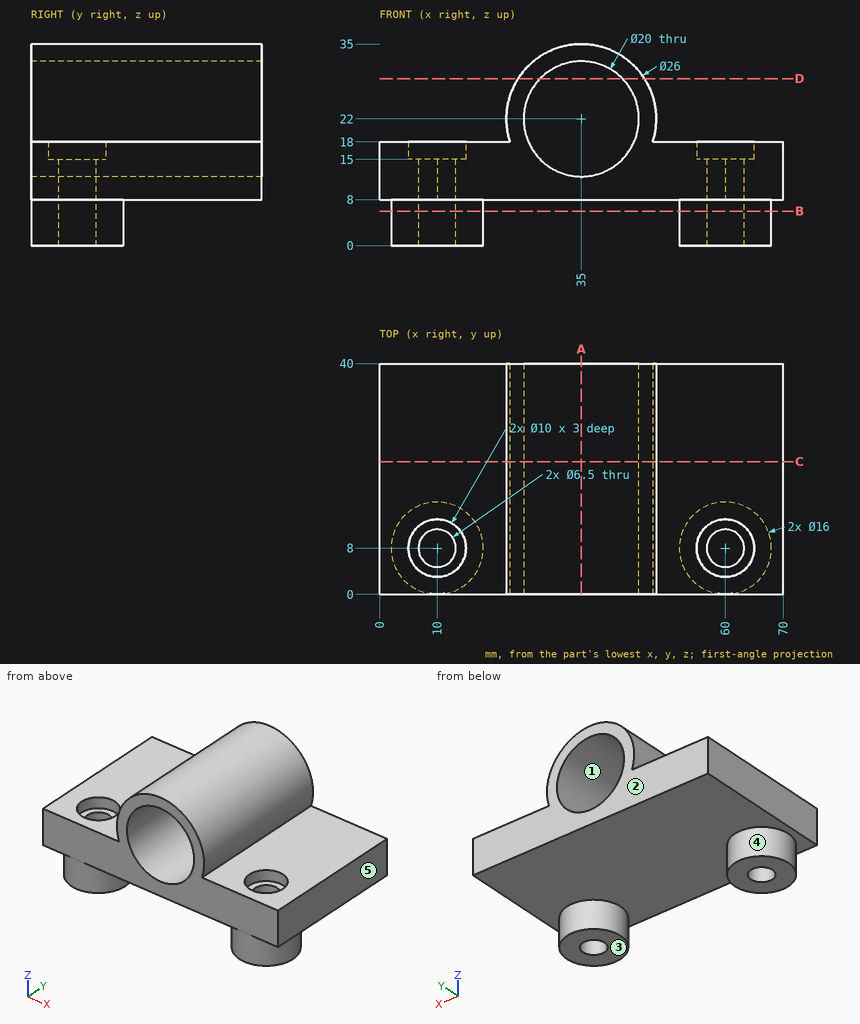
Job drawing, mm, ordinate dimensions from the low corner. One solid piece. A direction names the side the tool comes from. Round coordinates to 2 decimals unless told otherwise and drop trailing zeros. Loops run counter-clockwise (first coordinate to the right, second up) from the corner with the lowest first, then second, coordinate; pieces in that order, holes last. Notation, with made-up numbers: M 30.5,67 L 40.5,67 A9 ccw 40.5,81 Z; hole C -15,25 d4. An arc over 180 degrees is marked long. One line per question, with ' | ' between items. Start each with the question number.
Item 1: Cut at D-D, the plane z = 29. Write the cut outline in (x, y), plus the area to 3 significant figures.
Item 2: Cut at C-C, the plane y = 23. Write the cut outline in (x, z), plus the area to 3 significant figures.
Item 3: Cut at A-A, the plane x = 35. Write the cut outline in (y, z), plus the area to 3 significant figures.
Item 4: Cut at B-B, the plane z = 6. Write the cut outline in (x, y).
Item 5: Pin check, flat tips, straight feed: pin 1 Ø5 at (x, y) = (21, 19) entering from -Z; pin 2 Ø8.5 at (x, y) = (10, 8) entering from +Z; pin 3 Ø3 at (y, z) = (15, 28.5) entering from -X; pin 4 Ø6 at (x, y) = (60, 8) entering from +Z. Stop position of each tip, or through.
Item 6: Two-plate mould, pull along Z, no slides. Class the marked faces 1, 2 and 3: pulls with the +Z half, pulls with the -Z half, needs draft (parallel to the pull), parting line crosses it, or undercut.
Item 7: Wall check: line 1 (Z direction, x = 35, y = 10); line 2 (X direction, y = 8, z = 16.1); line 3 (Y direction, x = 60, z = 8.75). Give the ranges that are in metal, low to high.
Item 8: Which spindle directions (+Z, -Z, +X, -X, +Y, -Y) get a long thin tool onto all of the face, cutting with end or side? Do the marked faces 4 and 5. Say none if no direction does.
Responses:
1) outline: M 24.05,0 L 27.86,0 L 27.86,40 L 24.05,40 Z; M 42.14,0 L 45.95,0 L 45.95,40 L 42.14,40 Z | area: 305 mm²
2) outline: M 0,8 L 70,8 L 70,18 L 47.37,18 A13 ccw long 22.63,18 L 0,18 Z; hole C 35,22 d20 | area: 754 mm²
3) outline: M 0,8 L 40,8 L 40,12 L 0,12 Z; M 0,32 L 40,32 L 40,35 L 0,35 Z | area: 280 mm²
4) outline: C 10,8 d16; C 60,8 d16; hole C 10,8 d6.5; hole C 60,8 d6.5
5) pin 1: stops at z = 8 | pin 2: stops at z = 15 | pin 3: stops at x = 23 | pin 4: passes through
6) face 1: undercut | face 2: needs draft | face 3: pulls with the -Z half
7) line 1: z = 8 to 12, 32 to 35 | line 2: x = 0 to 5, 15 to 26.93, 43.07 to 55, 65 to 70 | line 3: y = 0 to 4.75, 11.25 to 40
8) face 4: -Z | face 5: +Z, -Z, +X, +Y, -Y
